Read the model definition and answer for the solid it produces. Units are mm, in the model's axes. Give positions to 0.01 mm unless a question says otherwise; leave off trailing zeros. Write each loop counter-clockwise with the first axis right and the second up, starting at its lowest first coordinate (ties: lowest second). Pieces come first, ordered by that corner, then holes. Notation, with made-up numbers: (17, -36) -> (55, -36) arc R9 ccw to (55, -20) -> close; hole circle Ø10 at (84, 40.25). An arc over 180 degrees is marked (long way). Put each result on its own line as item: value. Start each with the question number.
from build123d import *

# Parameters (mm, degrees)
SKETCH1_W           = 50.8
SKETCH1_H           = 50.8
BOSS_EXTRUDE1_DEPTH = 76.2
CUT_EXTRUDE1_DEPTH  = 76.2


with BuildPart() as part:
    # Sketch1 → Boss-Extrude1 (new body)
    with BuildSketch(Plane(origin=(0, 0, 0), x_dir=(0, 0, -1), z_dir=(1, 0, 0))):
        Rectangle(SKETCH1_W, SKETCH1_H)
    extrude(amount=BOSS_EXTRUDE1_DEPTH)

    # Sketch2 → Cut-Extrude1 (cut)
    with BuildSketch(Plane(origin=(76.2, 0, 0), x_dir=(0, 0, -1), z_dir=(1, 0, 0))):
        with BuildLine():
            Line((0, -25.4), (0, -23.4))
            ThreePointArc((0, -23.4), (16.54629868, -16.54629868), (23.4, 0))
            Line((23.4, 0), (25.4, 0))
            Line((25.4, 0), (25.4, 25.4))
            Line((25.4, 25.4), (-25.4, 25.4))
            Line((-25.4, 25.4), (-25.4, -25.4))
            Line((-25.4, -25.4), (0, -25.4))
        make_face()
    extrude(amount=-CUT_EXTRUDE1_DEPTH, mode=Mode.SUBTRACT)


solid = part.part
1) A cutting plane is placed at C-C on z = -21. Give the vertices of the cut face in (x, y), and give its area (3 significant figures).
2) Each of these flat-tipped pins is pushed along its axis until it touches: pin 1 Ø2 at (x, z) = (20, -14.5) entering from +Y; pin 2 Ø5 at (y, z) = (-18, -9) entering from +X; pin 3 Ø12 at (x, y) = (40, -13) entering from +Z. Where does it stop, or does it pass through?
3) A cutting plane is placed at A-A on x = 63. Give the vertices of the cut face in (y, z).
4) A cutting plane is placed at B-B on y = -10. Give the vertices of the cut face in (x, z).
5) Straight lines are drawn through the part: line 1 (Z direction, x = 59, y = -4.75); line 2 (Y direction, x = 61.5, z = -6.25); line 3 (Z direction, x = 55, y = -10.5). For each, find the intervals that lie inside material, in ascending order. Write a range as [from, to].
6) For a pull along Y with two mould halves and no side action, classify faces 1 (the face through (38, -25.4, -13)), 2 (the face through (39, -24, 0)), 3 (the face through (39, 0, -24)) as pulls with the +Y half, pulls with the -Y half, needs draft (parallel to the pull), parting line crosses it, or undercut.
Results found:
1. outline: (0, -25.4) -> (76.2, -25.4) -> (76.2, -10.32) -> (0, -10.32) -> close
1. area: 1,150 mm²
2. pin 1: stops at y = -17.53
2. pin 2: passes through
2. pin 3: stops at z = -13.66
3. outline: (-25.4, -25.4) -> (0, -25.4) -> (0, -23.4) arc R23.4 cw to (-23.4, 0) -> (-25.4, 0) -> close
4. outline: (0, -25.4) -> (76.2, -25.4) -> (76.2, -21.16) -> (0, -21.16) -> close
5. line 1: z = [-25.4, -22.91]
5. line 2: y = [-25.4, -22.55]
5. line 3: z = [-25.4, -20.91]
6. face 1: pulls with the -Y half
6. face 2: needs draft
6. face 3: pulls with the +Y half
